from build123d import *

# Parameters (mm, degrees)
F0_W          = 3.175
F0_H          = 25.4
F1_DEPTH      = 19.05
F2_R          = 2.38125
F3_DEPTH      = 25.4
F4_W          = 3.175
F4_H          = 25.4
F5_DEPTH      = 20.574
F5_DEPTH_BACK = 1.5875


with BuildPart() as f1:
    # F0 (on Front) → F1 (new body)
    with BuildSketch(Plane.XZ):
        Rectangle(F0_W, F0_H)
    extrude(amount=F1_DEPTH)

    # F2 (on face) → F3 (cut)
    with BuildSketch(Plane.YZ.offset(1.5875)):
        with BuildLine():
            ThreePointArc((-19.05, 6.35), (-17.1901280605, 10.8401280605), (-12.7, 12.7))
            Line((-12.7, 12.7), (-19.05, 12.7))
            Line((-19.05, 12.7), (-19.05, 6.35))
        make_face()
        with BuildLine():
            ThreePointArc((-12.7, -12.7), (-17.1901280605, -10.8401280605), (-19.05, -6.35))
            Line((-19.05, -6.35), (-19.05, -12.7))
            Line((-19.05, -12.7), (-12.7, -12.7))
        make_face()
        with Locations((-9.212619625, 0)):
            Circle(F2_R)
    extrude(amount=-F3_DEPTH, mode=Mode.SUBTRACT)

    # F4 (on Right) → F5 (join, two sides)
    with BuildSketch(Plane.YZ) as f5_sk:
        with Locations((1.5875, 0)):
            Rectangle(F4_W, F4_H)
    extrude(amount=-F5_DEPTH)
    extrude(f5_sk.sketch, amount=F5_DEPTH_BACK)


solid = f1.part
Verification items for the finished model (mm, model axes). A direction names the side the tool comes from. Give positions to 0.01 mm unless a question says otherwise; leave off trailing zeros. Loops run counter-clockwise (first coordinate to the right, second up) from the corner with the lowest first, then second, coordinate; pieces in that order, holes last. Notation, with made-up numbers: (28, 72) - (72, 72) arc R38 ccw to (72, 110) - close; hole circle Ø2 at (10, 7). An arc over 180 degrees is marked (long way). Write item = value, one per line. Start each with the question number.
Q1. Mould release check, pull along Y, two halves, no side actions. Record for faces 3 (the face through (0.02, -17.24, 10.79)), 4 (the face through (0.02, -11.59, 0.1)), 5 (the face through (-10, 3.175, 0)): released by +Y, released by -Y, zero draft, split by the parting line, or undercut.
Q2. Cross-section at D-D, the plane x = -3.5. Enter the section's corners in (y, z) (3 decimals).
Q3. Depth check by flat-ended pin: P1, Ø1, axis at x = -15, z = 7, coming from the -Y side; P2, Ø4.5, axis at y = -9.21, z = 0, coming from the -X side; P3, Ø9.5, axis at y = -6.5, z = 0, coming from the -X side. Enter the tip coordinate at first touch or a pass-through.
Q4. Cross-section at B-B, the plane y = -9.5. Enter the section's corners in (x, z).
Q5. Tool access check on faces 1 (the face through (-11, 0, 0)), 2 (the face through (0.02, -17.14, -10.89)). Record the directions out of +Z, -Z, +X, -X, +Y, -Y that give a thin tool (end or side, any length) a straight path to the whole face; none if there is none.
Q6. Thickness scan on line 1 (X direction, y = -17, z = 4.5); line 2 (Y direction, x = -2.75, z = -4.25) (3 decimals); line 3 (Z direction, x = -0.5, y = -15). Record the ranges inside material, lowest first.
Answer key:
q1.face_3 = released by -Y
q1.face_4 = undercut
q1.face_5 = released by +Y
q2.outline = (0, -12.7) - (3.175, -12.7) - (3.175, 12.7) - (0, 12.7) - close
q3.P1 = 0
q3.P2 = through
q3.P3 = -1.59
q4.outline = (-1.59, -12.7) - (1.59, -12.7) - (1.59, -2.36) - (-1.59, -2.36) - close; (-1.59, 2.36) - (1.59, 2.36) - (1.59, 12.7) - (-1.59, 12.7) - close
q5.face_1 = +Z, -Z, -X, -Y
q5.face_2 = -Z, +X, -X, -Y
q6.line_1 = -1.59 to 1.59
q6.line_2 = 0 to 3.175
q6.line_3 = -12.27 to 12.27
